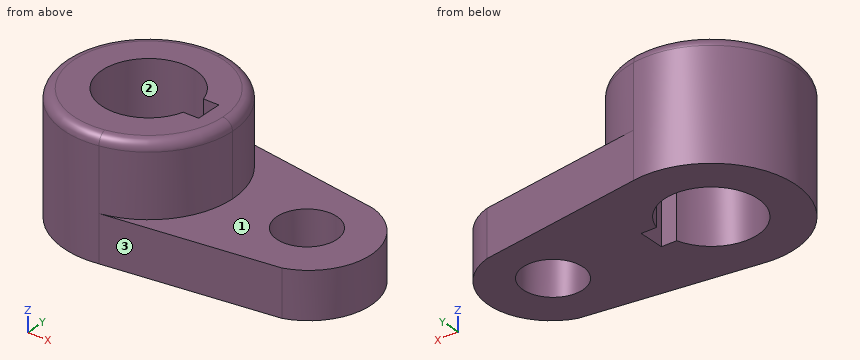
from build123d import *

# Parameters (mm, degrees)
F2_DEPTH = 40.2336
F3_DEPTH = 15.7734
F4_R     = 3.302
F1_R     = 10.16
F5_DEPTH = 40.64


with BuildPart() as f2:
    # F0 (on Top) → F2 (new body)
    with BuildSketch(Plane.XY):
        with BuildLine():
            ThreePointArc((4.744137, -28.178428), (21.818505, -18.452194), (28.575, 0))
            ThreePointArc((28.575, 0), (21.818505, 18.452194), (4.744137, 28.178428))
            ThreePointArc((4.744137, 28.178428), (-28.575, 0), (4.744137, -28.178428))
        make_face()
        with BuildLine():
            ThreePointArc((15.231124, -4.475321), (-15.875, -0.002348), (15.229799, 4.479826))
            Line((15.229799, 4.479826), (20.463184, 4.475321))
            Line((20.463184, 4.475321), (20.463184, -4.475321))
            Line((20.463184, -4.475321), (15.231124, -4.475321))
        make_face(mode=Mode.SUBTRACT)
    extrude(amount=F2_DEPTH)

    # F0 (on Top) → F3 (join)
    with BuildSketch(Plane.XY):
        with BuildLine():
            ThreePointArc((4.744137, 28.178428), (21.818505, 18.452194), (28.575, 0))
            ThreePointArc((28.575, 0), (21.818505, -18.452194), (4.744137, -28.178428))
            Line((4.744137, -28.178428), (61.701294, -21.083742))
            ThreePointArc((61.701294, -21.083742), (76.474609, -0.919848), (61.701294, 19.244047))
            Line((61.701294, 19.244047), (4.744137, 28.178428))
        make_face()
    extrude(amount=F3_DEPTH)

    # F4
    f4_edges = [f2.edges().sort_by_distance(p)[0] for p in [
        (-4.744137, 28.178428, 40.2336),
    ]]
    fillet(f4_edges, radius=F4_R)

    # F1 (on Top) → F5 (cut)
    with BuildSketch(Plane.XY):
        with Locations((53.975, 0)):
            Circle(F1_R)
    extrude(amount=F5_DEPTH, mode=Mode.SUBTRACT)


solid = f2.part
Read the model definition and answer for the solid it produces. Units are mm, in the model's axes. Face numbers are marked on the shaded views. Coordinates: 2 decimals unless noted, no trailing zeros. Loops run counter-clockwise (first coordinate to the right, second up) from the corner with the lowest first, then second, coordinate; pieces in that order, holes last. Notation, with made-up numbers: (-40, 86) -> (14, 86) arc R16 ccw to (14, 108) -> close; hole circle Ø3 at (56, 10.5). An arc over 180 degrees is marked (long way). Write item = value, one per line. Start each with the question number.
1) The part is cut by section B-B, the plane z = 32. Determine the outline of the cut face in (x, y) (3 decimals), plus the area to 3 significant figures.
2) The part is cut by section A-A, the plane z = 13.5. Determine the outline of the cut face in (x, y) (3 decimals), plus the area to 3 significant figures.
3) Find the intervals of material crossed by L1, parallel to Y at x = 0, z = 30 (3 decimals); L2, parallel to X at y = 7, z = 3; L3, parallel to Z at x = 33.5, y = 2, in increasing order. Write a range as from..to.
4) The mould has two halves that part along X. Classify the marked faces 1, 2 and 3: pulls with the +X half, pulls with the -X half, needs draft (parallel to the pull), parting line crosses it, or undercut.
5) The part is cut by section C-C, the plane y = -6.5. State how many separate pieces and enclosed holes the cut face has, plus the area to 3 significant figures.
6) Given P1, Ø12, axis at x = 27, z = 33, coming from the +Y side; P2, Ø2, axis at x = 5, z = 24.5, coming from the -Y side; P3, Ø16.5, axis at x = 53.975, y = 0, coming from the -Z side (1 decimal); P4, Ø1.6, axis at x = 17, z = 16.5, coming from the +Y side, each flat-ended and moving along its own axis, determine where each tip first touches the part or whether it passes through.
Result:
q1.outline = circle Ø57.15 at (0, 0); hole (15.23, 4.48) arc R15.875 ccw (long way) to (15.231, -4.475) -> (20.463, -4.475) -> (20.463, 4.475) -> close
q1.area = 1,730 mm²
q2.outline = (4.744, -28.178) -> (61.701, -21.084) arc R21.147 ccw to (61.701, 19.244) -> (4.744, 28.178) arc R28.575 ccw (long way) to start; hole (15.23, 4.48) arc R15.875 ccw (long way) to (15.231, -4.475) -> (20.463, -4.475) -> (20.463, 4.475) -> close; hole circle Ø20.32 at (53.975, 0)
q2.area = 3,580 mm²
q3.L1 = -28.575..-15.875, 15.875..28.575
q3.L2 = -27.7..-14.25, 14.25..46.61, 61.34..74.94
q3.L3 = 0..15.77
q4.face_1 = needs draft
q4.face_2 = undercut
q4.face_3 = pulls with the +X half
q5.separate_pieces = 3
q5.enclosed_holes = 0
q5.area = 1,580 mm²
q6.P1 = 19.38
q6.P2 = -28.29
q6.P3 = through
q6.P4 = 26.31
